Part model, mm, in its own coordinate system. A direction names the side the tool comes from. Give positions to 0.01 mm unless a question says otherwise; leave off trailing zeros. Write each loop counter-clockwise with the first axis right and the second up, starting at its lowest first coordinate (ties: lowest second). Pieces come first, ordered by that corner, then holes.
```python
from build123d import *

# Parameters (mm, degrees)
SKETCH1_W           = 30
SKETCH1_H           = 3
SKETCH1_W_2         = 7
SKETCH1_H_2         = 17
BOSS_EXTRUDE1_DEPTH = 15
BOSS_EXTRUDE2_DEPTH = 3
BOSS_EXTRUDE3_START = -15
BOSS_EXTRUDE3_DEPTH = 3
SKETCH4_R           = 2.5
CUT_EXTRUDE1_DEPTH  = 7
SKETCH5_R           = 2.25
CUT_EXTRUDE2_DEPTH  = 7
FILLET3_R           = 3
FILLET4_R           = 2


with BuildPart() as part:
    # Sketch1 → Boss-Extrude1 (new body)
    with BuildSketch(Plane(origin=(0, 0, 0), x_dir=(1, 0, 0), z_dir=(0, 1, 0))):
        Rectangle(SKETCH1_W, SKETCH1_H)
        with Locations((-11.5, 10)):
            Rectangle(SKETCH1_W_2, SKETCH1_H_2)
    extrude(amount=BOSS_EXTRUDE1_DEPTH)

    # Sketch3 → Boss-Extrude2 (add)
    with BuildSketch(Plane(origin=(0, 15, 0), x_dir=(1, 0, 0), z_dir=(0, 1, 0))):
        Polygon((-8, 18.5), (2, 1.5), (-8, 1.5), align=None)
    extrude(amount=-BOSS_EXTRUDE2_DEPTH)

    # Sketch3<3> → Boss-Extrude3 (add)
    with BuildSketch(Plane(origin=(0, 15, 0), x_dir=(1, 0, 0), z_dir=(0, 1, 0)).offset(BOSS_EXTRUDE3_START)):
        Polygon((-8, 18.5), (2, 1.5), (-8, 1.5), align=None)
    extrude(amount=BOSS_EXTRUDE3_DEPTH)

    # Sketch4 → Cut-Extrude1 (cut)
    with BuildSketch(Plane.ZY.offset(15)):
        with Locations((-3.5, 11)):
            Circle(SKETCH4_R)
        with Locations((-13.5, 11)):
            Circle(SKETCH4_R)
        with Locations((-3.5, 4)):
            Circle(SKETCH4_R)
        with Locations((-13.5, 4)):
            Circle(SKETCH4_R)
    extrude(amount=-CUT_EXTRUDE1_DEPTH, mode=Mode.SUBTRACT)

    # Sketch5 → Cut-Extrude2 (cut)
    with BuildSketch(Plane(origin=(0, 0, -1.5), x_dir=(-1, 0, 0), z_dir=(0, 0, -1))):
        with Locations((-9, 7.5)):
            Circle(SKETCH5_R)
        with Locations((4, 7.5)):
            Circle(SKETCH5_R)
    extrude(amount=-CUT_EXTRUDE2_DEPTH, mode=Mode.SUBTRACT)

    # Fillet3
    fillet3_edges = [part.edges().sort_by_distance(p)[0] for p in [
        (15, 15, 0),
        (15, 0, 0),
    ]]
    fillet(fillet3_edges, radius=FILLET3_R)

    # Fillet4
    fillet4_edges = [part.edges().sort_by_distance(p)[0] for p in [
        (-11.5, 15, -18.5),
        (-11.5, 0, -18.5),
    ]]
    fillet(fillet4_edges, radius=FILLET4_R)


solid = part.part
```
1) Saw through at C-C, the plane z = -0.5. Write the cut outline in (x, y), then the cut area to 3 significant figures.
Answers follow:
outline: (-15, 0) - (12, 0) arc R3 ccw to (15, 3) - (15, 12) arc R3 ccw to (12, 15) - (-15, 15) - close; hole circle Ø4.5 at (-4, 7.5); hole circle Ø4.5 at (9, 7.5)
area: 414 mm2
2) Two-plate mould, pull along Y, no slides. Class faces 1 (the face through (-8, 13, -3)), 2 (the face through (-8, 13, -14)), 3 (the face through (-10.85, 14.43, -17.9)), 4 (the face through (0, 7, 1.5)): +Y half, -Y half, draft (parallel to the pull), parting line (faces both ways), or undercut.
Answers follow:
face 1: undercut
face 2: undercut
face 3: +Y half
face 4: draft
3) Saw through at A-A, the plane y = 4. Write the cut outline in (x, z), then the cut area to 3 significant figures.
Answers follow:
outline: (-15, -18.5) - (-8, -18.5) - (-8, -16) - (-15, -16) - close; (-15, -11) - (-8, -11) - (-8, -6) - (-15, -6) - close; (-15, -1) - (-8, -1) - (-8, -1.5) - (15, -1.5) - (15, 1.5) - (-15, 1.5) - close
area: 139 mm2
4) Saw through at D-D, the plane z = -13.5. Write the cut outline in (x, y), then the cut area to 3 significant figures.
Answers follow:
outline: (-15, 0) - (-5.06, 0) - (-5.06, 3) - (-8, 3) - (-8, 1.5) - (-15, 1.5) - close; (-15, 6.5) - (-8, 6.5) - (-8, 8.5) - (-15, 8.5) - close; (-15, 13.5) - (-8, 13.5) - (-8, 12) - (-5.06, 12) - (-5.06, 15) - (-15, 15) - close
area: 52.6 mm2
5) Pin check, flat tips, straight feed: pin 1 Ø3 at (y, z) = (4, -3.5) entering from +X; pin 2 Ø1 at (x, y) = (0.5, 12) entering from -Z; pin 3 Ø4 at (x, y) = (-6, 7.5) entering from +Z; pin 4 Ø1.2 at (y, z) = (2.5, -13) entering from -X. Stop position of each tip, or through.
Answers follow:
pin 1: stops at x = 1.48
pin 2: stops at z = -4.9
pin 3: stops at z = 1.5
pin 4: stops at x = -8
6) 3-axis set-ups, long thin cutter, end or side, ignore diameter. For faces 5 (the face through (-5, 12, -6)), 6 (the face through (-12, 7, -18.5)), 7 (the face through (-11.549, 4.751, -1.115)): which of +Z, -Z, +X, -X, +Y, -Y reach the whole face in a straight line?
Answers follow:
face 5: -Z, +X
face 6: -Z, +X, -X, +Y, -Y
face 7: -X
7) Wall check: L1, parallel to Y at x = -11.25, z = -13.5; L2, parallel to Z at x = -12.5, y = 4; L3, parallel to Y at x = -10, z = -12.25. Give the ranges that are in metal, low to high.
Answers follow:
L1: y = 0 to 1.5, 6.5 to 8.5, 13.5 to 15
L2: z = -18.5 to -16, -11 to -6, -1 to 1.5
L3: y = 0 to 1.83, 6.17 to 8.83, 13.17 to 15
8) Saw through at B-B, the plane x = -4. Write the cut outline in (y, z).
Answers follow:
outline: (0, -11.7) - (3, -11.7) - (3, -1.5) - (5.25, -1.5) - (5.25, 1.5) - (0, 1.5) - close; (9.75, -1.5) - (12, -1.5) - (12, -11.7) - (15, -11.7) - (15, 1.5) - (9.75, 1.5) - close
